Can you work these out from the model? Positions are in its coordinate system, mm. Round coordinates to 2 decimals unless told otherwise and drop trailing zeros. Loops run counter-clockwise (first coordinate to the right, second up) from the corner with the lowest first, then second, coordinate; pieces in that order, holes last.
from build123d import *

# Parameters (mm, degrees)
SKETCH1_W           = 37.9349
SKETCH1_H           = 37.9349
BOSS_EXTRUDE1_DEPTH = 3.175
SKETCH9_R           = 1.1176
CUT_EXTRUDE2_DEPTH  = 3.175
SKETCH12_W          = 3.3274
SKETCH12_H          = 4.5466
CUT_EXTRUDE4_DEPTH  = 3.175
SKETCH15_W          = 3.3528
SKETCH15_H          = 4.5212
CUT_EXTRUDE3_DEPTH  = 3.175
SKETCH13_W          = 10.16
SKETCH13_H          = 4.7117
CUT_EXTRUDE5_DEPTH  = 3.175
SKETCH14_W          = 4.8006
SKETCH14_H          = 6.0833
CUT_EXTRUDE6_DEPTH  = 3.175


with BuildPart() as part:
    # Sketch1 → Boss-Extrude1 (new body)
    with BuildSketch(Plane.XY):
        with Locations((18.96745, 18.96745)):
            Rectangle(SKETCH1_W, SKETCH1_H)
    extrude(amount=BOSS_EXTRUDE1_DEPTH)

    # Sketch9 → Cut-Extrude2 (cut)
    with BuildSketch(Plane.XY.offset(3.175)):
        with Locations((33.62325, 33.62325)):
            Circle(SKETCH9_R)
        with Locations((4.31165, 33.62325)):
            Circle(SKETCH9_R)
        with Locations((4.31165, 4.31165)):
            Circle(SKETCH9_R)
        with Locations((33.62325, 4.31165)):
            Circle(SKETCH9_R)
        with BuildLine():
            Line((35.385619933, 12.100169933), (35.385619933, 2.549280067))
            Line((35.385619933, 2.549280067), (25.834730067, 2.549280067))
            ThreePointArc((25.834730067, 2.549280067), (25.2984, 2.01295), (25.834730067, 1.476619933))
            Line((25.834730067, 1.476619933), (35.385619933, 1.476619933))
            ThreePointArc((35.385619933, 1.476619933), (37.303202335, 0.631697665), (36.458280067, 2.549280067))
            Line((36.458280067, 2.549280067), (36.458280067, 12.100169933))
            ThreePointArc((36.458280067, 12.100169933), (35.92195, 12.6365), (35.385619933, 12.100169933))
        make_face()
        with BuildLine():
            Line((35.385619933, 36.458280067), (25.834730067, 36.458280067))
            ThreePointArc((25.834730067, 36.458280067), (25.2984, 35.92195), (25.834730067, 35.385619933))
            Line((25.834730067, 35.385619933), (35.385619933, 35.385619933))
            Line((35.385619933, 35.385619933), (35.385619933, 25.834730067))
            ThreePointArc((35.385619933, 25.834730067), (35.92195, 25.2984), (36.458280067, 25.834730067))
            Line((36.458280067, 25.834730067), (36.458280067, 35.385619933))
            ThreePointArc((36.458280067, 35.385619933), (37.303202335, 37.303202335), (35.385619933, 36.458280067))
        make_face()
        with BuildLine():
            Line((12.048880067, 36.458280067), (2.549280067, 36.458280067))
            ThreePointArc((2.549280067, 36.458280067), (0.631697665, 37.303202335), (1.476619933, 35.385619933))
            Line((1.476619933, 35.385619933), (1.476619933, 25.886019933))
            ThreePointArc((1.476619933, 25.886019933), (2.01295, 25.349689867), (2.549280067, 25.886019933))
            Line((2.549280067, 25.886019933), (2.549280067, 35.385619933))
            Line((2.549280067, 35.385619933), (12.048880067, 35.385619933))
            ThreePointArc((12.048880067, 35.385619933), (12.585210133, 35.92195), (12.048880067, 36.458280067))
        make_face()
        with BuildLine():
            Line((23.06955, 36.458280067), (14.86535, 36.458280067))
            ThreePointArc((14.86535, 36.458280067), (14.329019933, 35.92195), (14.86535, 35.385619933))
            Line((14.86535, 35.385619933), (23.06955, 35.385619933))
            ThreePointArc((23.06955, 35.385619933), (23.605880067, 35.92195), (23.06955, 36.458280067))
        make_face()
        with BuildLine():
            Line((2.549280067, 23.06955), (2.549280067, 14.86535))
            ThreePointArc((2.549280067, 14.86535), (2.01295, 14.329019933), (1.476619933, 14.86535))
            Line((1.476619933, 14.86535), (1.476619933, 23.06955))
            ThreePointArc((1.476619933, 23.06955), (2.01295, 23.605880067), (2.549280067, 23.06955))
        make_face()
        with BuildLine():
            Line((36.458280067, 23.06955), (36.458280067, 14.86535))
            ThreePointArc((36.458280067, 14.86535), (35.92195, 14.329019933), (35.385619933, 14.86535))
            Line((35.385619933, 14.86535), (35.385619933, 23.06955))
            ThreePointArc((35.385619933, 23.06955), (35.92195, 23.605880067), (36.458280067, 23.06955))
        make_face()
        with BuildLine():
            Line((23.06955, 2.549280067), (14.86535, 2.549280067))
            ThreePointArc((14.86535, 2.549280067), (14.329019933, 2.01295), (14.86535, 1.476619933))
            Line((14.86535, 1.476619933), (23.06955, 1.476619933))
            ThreePointArc((23.06955, 1.476619933), (23.605880067, 2.01295), (23.06955, 2.549280067))
        make_face()
        with BuildLine():
            Line((2.549280067, 12.100169933), (2.549280067, 2.549280067))
            Line((2.549280067, 2.549280067), (12.100169933, 2.549280067))
            ThreePointArc((12.100169933, 2.549280067), (12.6365, 2.01295), (12.100169933, 1.476619933))
            Line((12.100169933, 1.476619933), (2.600569933, 1.476619933))
            ThreePointArc((2.600569933, 1.476619933), (0.681867267, 0.681867267), (1.476619933, 2.600569933))
            Line((1.476619933, 2.600569933), (1.476619933, 12.100169933))
            ThreePointArc((1.476619933, 12.100169933), (2.01295, 12.6365), (2.549280067, 12.100169933))
        make_face()
    extrude(amount=-CUT_EXTRUDE2_DEPTH, mode=Mode.SUBTRACT)

    # Sketch12 → Cut-Extrude4 (cut)
    with BuildSketch(Plane(origin=(0, 0, 0), x_dir=(-1, 0, 0), z_dir=(0, 0, -1))):
        with Locations((-33.721919933, 18.96745)):
            Rectangle(SKETCH12_W, SKETCH12_H)
    extrude(amount=-CUT_EXTRUDE4_DEPTH, mode=Mode.SUBTRACT)

    # Sketch15 → Cut-Extrude3 (cut)
    with BuildSketch(Plane(origin=(0, 0, 0), x_dir=(-1, 0, 0), z_dir=(0, 0, -1))):
        with Locations((-4.225680067, 17.3228)):
            Rectangle(SKETCH15_W, SKETCH15_H)
    extrude(amount=-CUT_EXTRUDE3_DEPTH, mode=Mode.SUBTRACT)

    # Sketch13 → Cut-Extrude5 (cut)
    with BuildSketch(Plane(origin=(0, 0, 0), x_dir=(-1, 0, 0), z_dir=(0, 0, -1))):
        with Locations((-23.8125, 4.905130067)):
            Rectangle(SKETCH13_W, SKETCH13_H)
    extrude(amount=-CUT_EXTRUDE5_DEPTH, mode=Mode.SUBTRACT)

    # Sketch14 → Cut-Extrude6 (cut)
    with BuildSketch(Plane(origin=(0, 0, 0), x_dir=(-1, 0, 0), z_dir=(0, 0, -1))):
        with Locations((-4.949580067, 12.02055)):
            Rectangle(SKETCH14_W, SKETCH14_H)
    extrude(amount=-CUT_EXTRUDE6_DEPTH, mode=Mode.SUBTRACT)


solid = part.part
(1) If we section it at D-D, the plane z = 0.45: State how many separate pieces and enclosed holes the cut face has, then the cut area to 3 significant figures.
Worked answers:
separate pieces: 1
enclosed holes: 10
area: 1,170 mm2
(2) If we section it at A-A, the plane y = 6.5: List the corners of the cut face in (x, z) for me (1 decimal).
Worked answers:
outline: (0, 0) - (1.5, 0) - (1.5, 3.2) - (0, 3.2) - close; (2.5, 0) - (18.7, 0) - (18.7, 3.2) - (2.5, 3.2) - close; (28.9, 0) - (35.4, 0) - (35.4, 3.2) - (28.9, 3.2) - close; (36.5, 0) - (37.9, 0) - (37.9, 3.2) - (36.5, 3.2) - close
(3) If we section it at B-B, the plane x = 31: List the corners of the cut face in (y, z) for me (3 decimals).
Worked answers:
outline: (0, 0) - (1.477, 0) - (1.477, 3.175) - (0, 3.175) - close; (2.549, 0) - (35.386, 0) - (35.386, 3.175) - (2.549, 3.175) - close; (36.458, 0) - (37.935, 0) - (37.935, 3.175) - (36.458, 3.175) - close
(4) If I drill on line 1 (X direction, y = 21, z = 0.7); line 2 (Y direction, x = 16.5, z = 2.3), over which ranges is the centre line in solid material (lowest first)?
Worked answers:
line 1: x = 0 to 1.48, 2.55 to 32.06, 36.46 to 37.93
line 2: y = 0 to 1.48, 2.55 to 35.39, 36.46 to 37.93
(5) If we mould it in two halves opening along X, with no side actions, what happens to faces 1 (the flat face through (19, 19, 0)), 2 (the cylindrical face through (35.91, 23.606, 1.61))? For each: released by +X, released by -X, zero draft, split by the parting line, or undercut.
Worked answers:
face 1: zero draft
face 2: undercut
(6) Will this pin go through, and if not, where does the flat tip stop? P1, Ø1.3, axis at x = 33.62, y = 33.62, coming from the -Z side.
Worked answers:
P1: passes through
